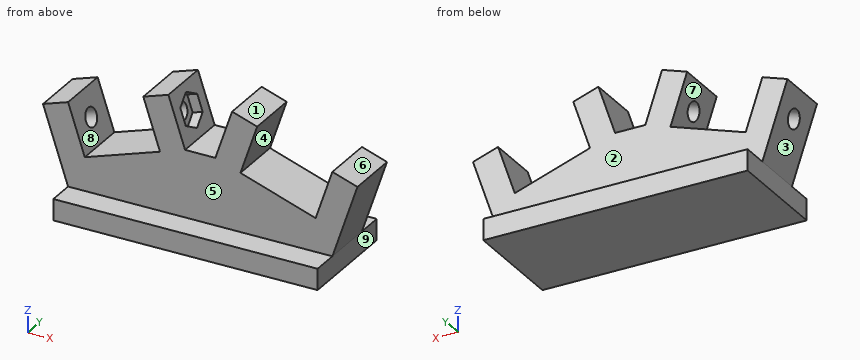
```python
from build123d import *

# Parameters (mm, degrees)
F0_W      = 50
F0_H      = 20
F1_DEPTH  = 4
F4_DEPTH  = 5
F5_R      = 1.75
F6_DEPTH  = 25
F8_DEPTH  = 2
F10_DEPTH = 10
F12_DEPTH = 10


with BuildPart() as f1:
    # F0 (on Top) → F1 (new body)
    with BuildSketch(Plane.XY):
        with Locations((25, 10)):
            Rectangle(F0_W, F0_H)
    extrude(amount=F1_DEPTH)

    # F3 (on offset) → F4 (join, symmetric)
    with BuildSketch(Plane.XZ.offset(-10)):
        Polygon((-4.7434164903, 18.2302494708), (0, 4), (5.2704627669, 4), (0, 19.8113883008), align=None)
        Polygon((14.2302494708, 24.5548047911), (21.0818510678, 4), (28.9181489322, 4), (35.7697505292, 24.5548047911), (31.026334039, 26.1359436212), (25, 8.0569415042), (18.973665961, 26.1359436212), align=None)
        Polygon((50, 4), (54.7434164903, 18.2302494708), (50, 19.8113883008), (44.7295372331, 4), align=None)
    extrude(amount=F4_DEPTH, both=True)

    # F5 (on face) → F6 (cut, through all)
    with BuildSketch(Plane(origin=(1.2, 0, 0.4), x_dir=(0, -1, 0), z_dir=(-0.9486832981, 0, -0.316227766))):
        with Locations((-10, 13.7947331922)):
            Circle(F5_R)
    extrude(amount=-F6_DEPTH, mode=Mode.SUBTRACT)

    # F7 (on face) → F8 (cut)
    with BuildSketch(Plane(origin=(24.9170824513, 0, 8.3056941504), x_dir=(0, 1, 0), z_dir=(0.9486832981, 0, 0.316227766))):
        Polygon((12.85, 12.1492849251), (12.85, 15.4401814595), (10, 17.0856297267), (7.15, 15.4401814595), (7.15, 12.1492849251), (10, 10.5038366579), align=None)
    extrude(amount=-F8_DEPTH, mode=Mode.SUBTRACT)

    # F9 (on face) → F10 (join, through all)
    with BuildSketch(Plane.XZ.offset(-5)):
        Polygon((22.135944317, 16.6491085532), (25, 8.0569415042), (27.864055683, 16.6491085532), align=None)
    extrude(amount=-F10_DEPTH)

    # F11 (on face) → F12 (join, through all)
    with BuildSketch(Plane.XZ.offset(-5)):
        Polygon((17.3925278267, 15.0679697232), (3.162278356, 10.3245532329), (5.2704627669, 4), (21.0818510678, 4), align=None)
        Polygon((28.9181489322, 4), (44.7295372331, 4), (46.837721644, 10.3245532329), (32.6074721733, 15.0679697232), align=None)
    extrude(amount=-F12_DEPTH)


solid = f1.part
```
The listing builds one solid part. Answer for the finished solid, in the listing's coordinates (mm). Face numbers are marked on the shaded views. A direction names the side the tool comes from. Round coordinates to 2 decimals unless told otherwise and drop trailing zeros. Loops run counter-clockwise (first coordinate to the right, second up) from the corner with the lowest first, then second, coordinate; pieces in that order, holes last.
1) For a pull along Z with two mould halves and no side action, classify the marked faces 1, 2, 3 and 4 as released by +Z, released by -Z, zero draft, split by the parting line, or undercut.
Outcome:
face 1: released by +Z
face 2: zero draft
face 3: released by -Z
face 4: undercut
2) Given P1, Ø2, axis at y = 10, z = 23, coming from the +X side; P2, Ø1.2, axis at y = 7.5, z = 1, coming from the +X side; P3, Ø3, axis at x = 19.5, z = 21, coming from the -Y side; P4, Ø1, axis at y = 3.5, z = 17, coming from the +X side, each flat-ended and moving along its own axis, determine where each tip first touches the part or whether it passes through.
Outcome:
P1: stops at x = 35.58
P2: stops at x = 50
P3: stops at y = 5
P4: passes through
3) A cutting plane is placed at A-A on y = 9.25. Give the number of separate pieces and of enclosed holes in the cut face, plus the area to 3 significant figures.
Outcome:
separate pieces: 3
enclosed holes: 0
area: 841 mm2
4) Consider line 1 (Z direction, x = 33, y = 16); line 2 (Y direction, x = 30.5, z = 16); line 3 (X direction, y = 17.75, z = 3.75). Determine where each line is inside the solid, lowest interval first.
Outcome:
line 1: z = 0 to 4
line 2: y = 5 to 15
line 3: x = 0 to 50
5) For the marked faces 5, 6, 7, 8 and 9, determine the directions among +Z, -Z, +X, -X, +Y, -Y from which every point of the face is accessible in a straight line to the end or side of a thin tool.
Outcome:
face 5: +Z, +X, -X, -Y
face 6: +Z, +X, +Y, -Y
face 7: +Y, -Y
face 8: +Z, +Y, -Y
face 9: -Z, +X, +Y, -Y
6) A cutting plane is placed at D-D on z = 5. Determine the outline of the cut face in (x, y).
Outcome:
outline: (-0.33, 5) - (50.33, 5) - (50.33, 15) - (-0.33, 15) - close
7) A cutting plane is placed at B-B on x = 29. Determine the outline of the cut face in (y, z).
Outcome:
outline: (0, 0) - (20, 0) - (20, 4) - (15, 4) - (15, 20.06) - (5, 20.06) - (5, 4) - (0, 4) - close
8) A cutting plane is placed at C-C on y = 2.75. Determine the outline of the cut face in (x, z), plus the area to 3 significant figures.
Outcome:
outline: (0, 0) - (50, 0) - (50, 4) - (0, 4) - close
area: 200 mm2
